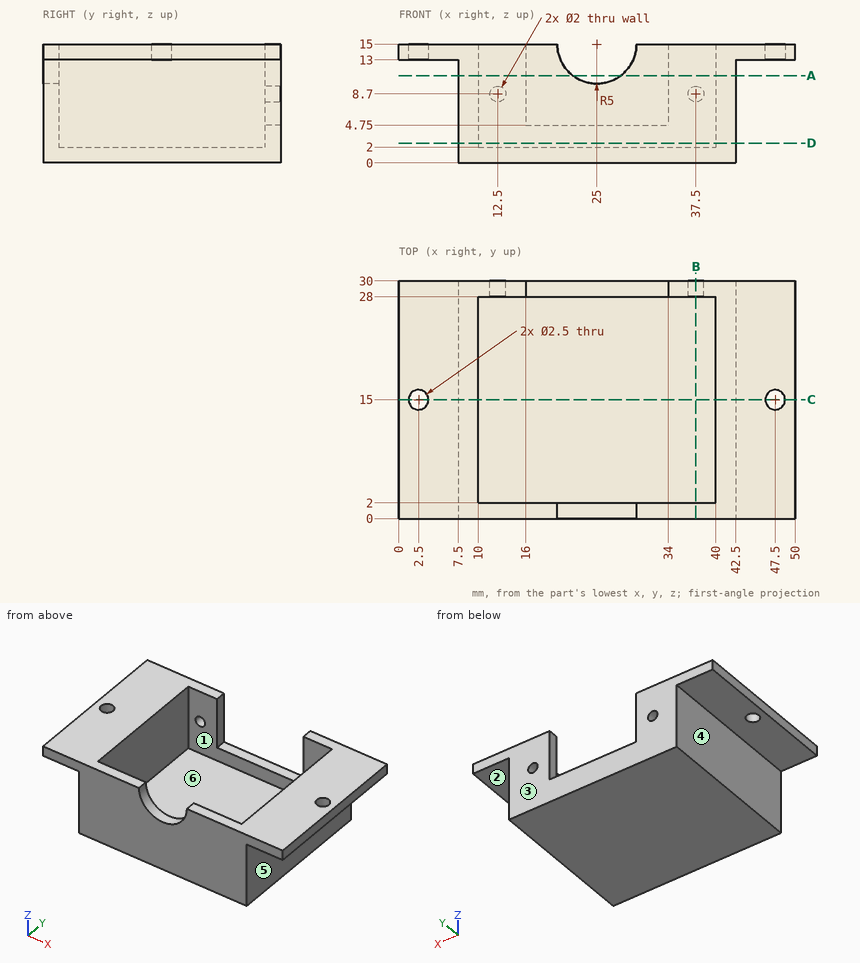
Can you work these out from the drawing? Everything is in mm from the part's minimum corner. A direction names the side the tool comes from. Give positions to 0.01 mm unless a question says otherwise; leave off trailing zeros. Order: outer loops, then holes, each group sorted by start corner. A loop starts at its lowest first (then second) coordinate and runs counter-clockwise, first axis right, second up.
1. For the marked faces 4, 5 and 6, which set-ups out of +Z, -Z, +X, -X, +Y, -Y let a thin tool reach every point of the face, with its end or its side?
2. We'd pull the mould along Y, two halves only. Please class the marked faces 1, 2 and 3: pulls with the +Y half, pulls with the -Y half, needs draft (parallel to the pull), parting line crosses it, or undercut.
3. Suppose I cut it at A-A (z = 11). List the corners of the cut face in (x, y) for me.
4. Suppose I cut it at C-C (y = 15). List the corners of the cut face in (x, z) for me.
5. Will these pins go through, and if not, where does the flat tip stop? P1, Ø2, axis at x = 4.5, y = 22, coming from the -Z side; P2, Ø1.6, axis at y = 29.5, z = 11.5, coming from the +X side; P3, Ø1.6, axis at x = 25, y = 29, coming from the +Z side.
6. Suppose I cut it at B-B (x = 37.5). List the corners of the cut face in (y, z) for me, plus the area to 3 significant figures.
7. I need wall thicknesses on L1, parallel to X at y = 29.55, z = 8.7; L2, parallel to Y at x = 47.5, z = 14.05; L3, parallel to X at y = 5.25, z = 14. Which ranges of each line are inside material? Lowest first, please.
8. Suppose I cut it at D-D (z = 2.5). List the corners of the cut face in (x, y) for me.
Solved:
1. face 4: -Z, -X, +Y, -Y
1. face 5: -Z, +X, +Y, -Y
1. face 6: +Z
2. face 1: undercut
2. face 2: needs draft
2. face 3: pulls with the +Y half
3. outline: (7.5, 0) - (22, 0) - (22, 2) - (10, 2) - (10, 28) - (16, 28) - (16, 30) - (7.5, 30) - close; (28, 0) - (42.5, 0) - (42.5, 30) - (34, 30) - (34, 28) - (40, 28) - (40, 2) - (28, 2) - close
4. outline: (0, 13) - (1.25, 13) - (1.25, 15) - (0, 15) - close; (3.75, 13) - (7.5, 13) - (7.5, 0) - (42.5, 0) - (42.5, 13) - (46.25, 13) - (46.25, 15) - (40, 15) - (40, 2) - (10, 2) - (10, 15) - (3.75, 15) - close; (48.75, 13) - (50, 13) - (50, 15) - (48.75, 15) - close
5. P1: stops at z = 13
5. P2: stops at x = 42.5
5. P3: stops at z = 4.75
6. outline: (0, 0) - (30, 0) - (30, 7.7) - (28, 7.7) - (28, 2) - (2, 2) - (2, 15) - (0, 15) - close; (28, 9.7) - (30, 9.7) - (30, 15) - (28, 15) - close
6. area: 108 mm2
7. L1: x = 7.5 to 11.5, 13.5 to 16, 34 to 36.5, 38.5 to 42.5
7. L2: y = 0 to 13.75, 16.25 to 30
7. L3: x = 0 to 10, 40 to 50
8. outline: (7.5, 0) - (42.5, 0) - (42.5, 30) - (7.5, 30) - close; hole (10, 2) - (40, 2) - (40, 28) - (10, 28) - close
